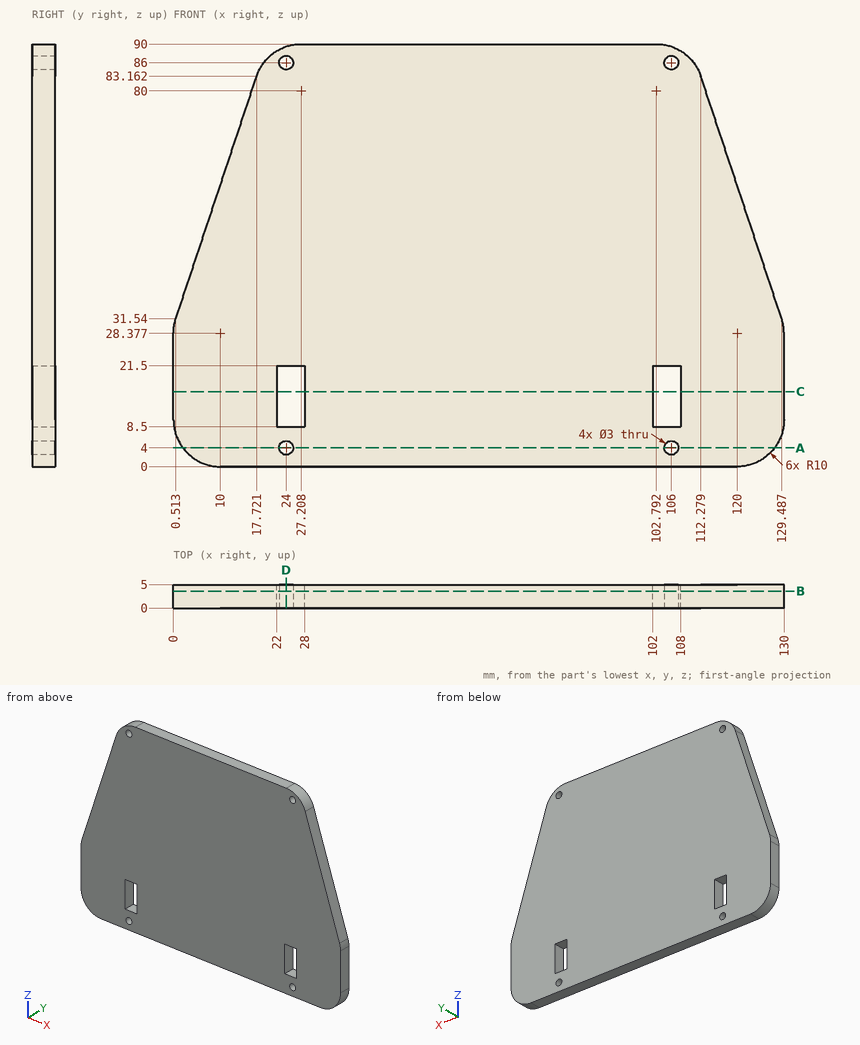
Check sheet for the drawn part. Datum: minimum x, y, z corner. Units: mm. Give positions to 0.01 mm unless a question says otherwise; leave off trailing zeros. Order: outer loops, then holes, each group sorted by start corner. A loop starts at its lowest first (then second) coordinate and runs counter-clockwise, first axis right, second up. Notation, with made-up numbers: (11, 78.5) -> (16, 78.5) arc R17 cw to (16, 84.5) -> close; hole circle Ø9 at (-24.75, 87). An arc over 180 degrees is marked (long way). Answer as CSV lines item,"result".
Q1. Sectioned sample at B-B on y = 3.6. Record the cut outline in (x, z), plus the area to 3 significant figures.
Solutions:
outline,"(0, 10) arc R10 ccw to (10, 0) -> (120, 0) arc R10 ccw to (130, 10) -> (130, 28.38) arc R10 ccw to (129.49, 31.54) -> (112.28, 83.16) arc R10 ccw to (102.79, 90) -> (27.21, 90) arc R10 ccw to (17.72, 83.16) -> (0.51, 31.54) arc R10 ccw to (0, 28.38) -> close; hole (22, 8.5) -> (28, 8.5) -> (28, 21.5) -> (22, 21.5) -> close; hole circle Ø3 at (24, 4); hole circle Ø3 at (24, 86); hole (102, 8.5) -> (108, 8.5) -> (108, 21.5) -> (102, 21.5) -> close; hole circle Ø3 at (106, 4); hole circle Ø3 at (106, 86)"
area,"10,300 mm²"
Q2. Sectioned sample at C-C on z = 16. Record the cut outline in (x, y), plus the area to 3 significant figures.
Solutions:
outline,"(0, 0) -> (22, 0) -> (22, 5) -> (0, 5) -> close; (28, 0) -> (102, 0) -> (102, 5) -> (28, 5) -> close; (108, 0) -> (130, 0) -> (130, 5) -> (108, 5) -> close"
area,"590 mm²"
Q3. Sectioned sample at A-A on z = 4. Record the cut outline in (x, y), plus the area to 3 significant figures.
Solutions:
outline,"(2, 0) -> (22.5, 0) -> (22.5, 5) -> (2, 5) -> close; (25.5, 0) -> (104.5, 0) -> (104.5, 5) -> (25.5, 5) -> close; (107.5, 0) -> (128, 0) -> (128, 5) -> (107.5, 5) -> close"
area,"600 mm²"
Q4. Scan lines: probe 1 along X at (y, z) = (1.9, 13.5); probe 2 along X at (y, z) = (1.6, 86); probe 3 along X at (y, z) = (2.45, 60). Record each from-to range of solid material in increasing order.
Solutions:
probe 1,"x = 0 to 22, 28 to 102, 108 to 130"
probe 2,"x = 19.21 to 22.5, 25.5 to 104.5, 107.5 to 110.79"
probe 3,"x = 10 to 120"
Q5. Sectioned sample at D-D on x = 24. Record the cut outline in (y, z).
Solutions:
outline,"(0, 0) -> (5, 0) -> (5, 2.5) -> (0, 2.5) -> close; (0, 5.5) -> (5, 5.5) -> (5, 8.5) -> (0, 8.5) -> close; (0, 21.5) -> (5, 21.5) -> (5, 84.5) -> (0, 84.5) -> close; (0, 87.5) -> (5, 87.5) -> (5, 89.47) -> (0, 89.47) -> close"
Q6. Depth check by flat-ended pin: pin 1 (2 mm diameter, centred on x = 105.5, y = 1.5, fed in from -Z); pin 2 (2.5 mm diameter, centred on x = 25, y = 2.5, fed in from +Z). Enter the tip coordinate at first touch or a pass-through.
Solutions:
pin 1,"stops at z = 0"
pin 2,"stops at z = 89.95"
